Source: CAD feature listing. Evaluate the final solid. Frame: model axes, mm. A direction names the side the tool comes from. Give positions to 0.01 mm unless a question says otherwise; leave off trailing zeros. Write each loop counter-clockwise with the first axis right and the second up, starting at its lowest first coordinate (ties: lowest second). Pieces come first, ordered by that corner, then holes.
```python
from build123d import *

# Parameters (mm, degrees)
F0_W     = 17.78
F0_H     = 17.78
F0_R     = 1.905
F1_DEPTH = 2.54
F3_DEPTH = 12.7
F4_R     = 1.905
F5_DEPTH = 25.4
F6_R     = 1.905
F7_DEPTH = 25.4
F8_DEPTH = 2.54


with BuildPart() as f1:
    # F0 (on Top) → F1 (new body)
    with BuildSketch(Plane.XY):
        with Locations((8.89, 8.89)):
            Rectangle(F0_W, F0_H)
        with Locations((9.7028, 9.7028)):
            Circle(F0_R, mode=Mode.SUBTRACT)
    extrude(amount=F1_DEPTH)

    # F2 (on face) → F3 (join)
    with BuildSketch(Plane.XY.offset(2.54)):
        Polygon((2.6436052285, 17.78), (0, 17.78), (0, 0), (17.78, 0), (17.78, 2.6436052285), (2.6436052285, 2.6436052285), align=None)
    extrude(amount=F3_DEPTH)

    # F4 (on face) → F5 (cut)
    with BuildSketch(Plane.XZ):
        with Locations((9.7028, 9.7028)):
            Circle(F4_R)
    extrude(amount=-F5_DEPTH, mode=Mode.SUBTRACT)

    # F6 (on face) → F7 (cut)
    with BuildSketch(Plane(origin=(0, 0, 0), x_dir=(0, -1, 0), z_dir=(-1, 0, 0))):
        with Locations((-9.7028, 9.7028)):
            Circle(F6_R)
    extrude(amount=-F7_DEPTH, mode=Mode.SUBTRACT)

    # F8 (add): a face of the model
    f8_faces = [f1.faces().sort_by_distance(p)[0] for p in [
        (2.3921580571, 10.2118026143, 15.24),
    ]]
    extrude(f8_faces, amount=F8_DEPTH)


solid = f1.part
```
1. Section query D-D (y = 2). Return loops of the section in (x, z) (3 decimals).
2. Section query B-B (z = 8.75). Return loops of the section in (x, y).
3. Pull-direction query (Z, two-part tool) for faces 1 (the cylindrical face through (11.46, 1.3, 8.97)), 2 (the flat face through (2, 6, 17.78)), 3 (the flat face through (12, 2.644, 10)); classes: pulls with the +Z half, pulls with the -Z half, needs draft (parallel to the pull), parting line crosses it, or undercut.
4. Section query C-C (z = 3.5). Return loops of the section in (x, y), plus the area to 3 significant figures.
5. Access query for faces 4 (the flat face through (2.644, 12, 10)), 5 (the cylindrical face through (1.303, 11.606, 9.787)). Directions: +Z, -Z, +X, -X, +Y, -Y. A direction counts if a zero-diameter tool reaches every point of the face in a straight line with its end or side. Return the directions, or none.
6. Pin query (flat end, axial travel): P1, Ø1.5, axis at x = 12.5, y = 6.5, coming from the -Z side; P2, Ø2, axis at y = 8, z = 14.5, coming from the +X side; P3, Ø4.5, axis at x = 9.7, z = 9.7, coming from the +Y side; P4, Ø2.5, axis at x = 9.7, y = 9.7, coming from the -Z side. Return the tip coordinate at first contact, or that it passes through.
7. Section query A-A (x = 11.25). Return loops of the section in (y, z).
8. Line query: probe 1 along Y at (x, z) = (4.5, 16.75); probe 2 along Z at (x, y) = (14.75, 2.75). Output: solid intervals per line, ascending.
The answers:
1. outline: (0, 0) - (17.78, 0) - (17.78, 17.78) - (0, 17.78) - close; hole circle Ø3.81 at (9.703, 9.703)
2. outline: (0, 0) - (8.05, 0) - (8.05, 2.64) - (2.64, 2.64) - (2.64, 8.05) - (0, 8.05) - close; (0, 11.35) - (2.64, 11.35) - (2.64, 17.78) - (0, 17.78) - close; (11.35, 0) - (17.78, 0) - (17.78, 2.64) - (11.35, 2.64) - close
3. face 1: undercut
3. face 2: pulls with the +Z half
3. face 3: needs draft
4. outline: (0, 0) - (17.78, 0) - (17.78, 2.64) - (2.64, 2.64) - (2.64, 17.78) - (0, 17.78) - close
4. area: 87.0 mm2
5. face 4: +Z, +X, +Y
5. face 5: +X, -X
6. P1: stops at z = 0
6. P2: stops at x = 2.64
6. P3: stops at y = 2.64
6. P4: passes through
7. outline: (0, 0) - (8.59, 0) - (8.59, 2.54) - (2.64, 2.54) - (2.64, 8.59) - (0, 8.59) - close; (0, 10.81) - (2.64, 10.81) - (2.64, 17.78) - (0, 17.78) - close; (10.81, 0) - (17.78, 0) - (17.78, 2.54) - (10.81, 2.54) - close
8. probe 1: y = 0 to 2.64
8. probe 2: z = 0 to 2.54
